from build123d import *

# Parameters (mm, degrees)
SKETCH1_W            = 13
SKETCH1_H            = 5.75
BOSS_EXTRUDE1_DEPTH  = 2.5
SKETCH2_W            = 0.75
SKETCH2_H            = 0.5
BOSS_EXTRUDE2_DEPTH  = 4
CHAMFER1_SIZE        = 0.2
SKETCH4_R            = 1
CUT_EXTRUDE1_DEPTH   = 6
SKETCH5_W            = 2
SKETCH5_H            = 0.2
BOSS_EXTRUDE3_DEPTH  = 5.75
CHAMFER2_SIZE        = 0.2
SKETCH10_W           = 13.0002
SKETCH10_H           = 5.7502
BOSS_EXTRUDE8_DEPTH  = 3.75
SKETCH11_W           = 3.5
SKETCH11_H           = 2.3
BOSS_EXTRUDE9_DEPTH  = 0.5
SKETCH12_W           = 3.5
SKETCH12_H           = 2.3
BOSS_EXTRUDE10_DEPTH = 0.5
SKETCH13_W           = 1
SKETCH13_H           = 2.5
BOSS_EXTRUDE11_DEPTH = 1
FILLET2_RADIUS       = 0.5
FILLET2_LENGTH       = 2.5
SKETCH14_W           = 5
SKETCH14_H           = 4.5
CUT_EXTRUDE2_DEPTH   = 0.05
SKETCH15_R           = 0.15
CUT_EXTRUDE3_DEPTH   = 10
SKETCH16_W           = 0.75
SKETCH16_H           = 4
CUT_EXTRUDE4_DEPTH   = 1.2


with BuildPart() as part:
    # Sketch1 → Boss-Extrude1 (new body)
    with BuildSketch(Plane.XY):
        Rectangle(SKETCH1_W, SKETCH1_H)
    extrude(amount=BOSS_EXTRUDE1_DEPTH)

    # Sketch2 → Boss-Extrude2 (add)
    with BuildSketch(Plane(origin=(0, 0, 0), x_dir=(-1, 0, 0), z_dir=(0, 0, -1))):
        Rectangle(SKETCH2_W, SKETCH2_H)
        with Locations((-5, 0)):
            Rectangle(SKETCH2_W, SKETCH2_H)
        with Locations((5, 0)):
            Rectangle(SKETCH2_W, SKETCH2_H)
    extrude(amount=BOSS_EXTRUDE2_DEPTH)

    # Chamfer1
    chamfer1_edges = [part.edges().sort_by_distance(p)[0] for p in [
        (-0.375, 0, -4),
        (0.375, 0, -4),
        (4.625, 0, -4),
        (5.375, 0, -4),
        (-5.375, 0, -4),
        (-4.625, 0, -4),
    ]]
    chamfer(chamfer1_edges, length=CHAMFER1_SIZE)

    # Sketch4 → Cut-Extrude1 (cut)
    with BuildSketch(Plane(origin=(0, 2.875, 0), x_dir=(1, 0, 0), z_dir=(0, 1, 0))):
        with Locations(Location((-3.25, -1.25, 0), (0, 0, 270))):
            Circle(SKETCH4_R)
        with Locations(Location((3.25, -1.25, 0), (0, 0, 270))):
            Circle(SKETCH4_R)
    extrude(amount=-CUT_EXTRUDE1_DEPTH, mode=Mode.SUBTRACT)

    # Sketch5 → Boss-Extrude3 (add)
    with BuildSketch(Plane(origin=(0, 2.875, 0), x_dir=(1, 0, 0), z_dir=(0, 1, 0))):
        with Locations((-3.25, 0.1)):
            Rectangle(SKETCH5_W, SKETCH5_H)
        with Locations((3.25, 0.1)):
            Rectangle(SKETCH5_W, SKETCH5_H)
    extrude(amount=-BOSS_EXTRUDE3_DEPTH)

    # Chamfer2
    chamfer2_edges = [part.edges().sort_by_distance(p)[0] for p in [
        (4.25, 0, 0),
        (2.25, 0, 0),
        (-2.25, 0, 0),
        (-4.25, 0, 0),
    ]]
    chamfer(chamfer2_edges, length=CHAMFER2_SIZE - 0.0001)  # a hair under: the kernel refuses the full size

    # Sketch10 → Boss-Extrude8 (add)
    with BuildSketch(Plane.XY.offset(2.5)):
        Rectangle(SKETCH10_W, SKETCH10_H)
    extrude(amount=BOSS_EXTRUDE8_DEPTH)

    # Sketch11 → Boss-Extrude9 (add)
    with BuildSketch(Plane.XZ.offset(2.8751)):
        with Locations((0, 1.35)):
            Rectangle(SKETCH11_W, SKETCH11_H)
    extrude(amount=-BOSS_EXTRUDE9_DEPTH)

    # Sketch12 → Boss-Extrude10 (add)
    with BuildSketch(Plane(origin=(0, 2.8751, 0), x_dir=(1, 0, 0), z_dir=(0, 1, 0))):
        with Locations((0, -1.35)):
            Rectangle(SKETCH12_W, SKETCH12_H)
    extrude(amount=-BOSS_EXTRUDE10_DEPTH)

    # Sketch13 → Boss-Extrude11 (add)
    with BuildSketch(Plane.XY.offset(6.25)):
        with Locations((-1.9999, 0)):
            Rectangle(SKETCH13_W, SKETCH13_H)
    extrude(amount=BOSS_EXTRUDE11_DEPTH)

    # Fillet2: full round fillet: the end face becomes a half cylinder, R = half its width
    fillet2_face = Plane((-1.9999, 0, 7.25), x_dir=(0, -1, 0), z_dir=(0, 0, 1))  # on the end face: x along it, z out of the body
    fillet2_slab = fillet2_face.offset(-FILLET2_RADIUS / 2) * Box(FILLET2_LENGTH, 2 * FILLET2_RADIUS, FILLET2_RADIUS, mode=Mode.PRIVATE)  # the body's end, R deep
    fillet2_round = Plane((-1.9999, 0, 6.75), x_dir=(0, 0, 1), z_dir=(0, -1, 0)) * Cylinder(FILLET2_RADIUS, FILLET2_LENGTH, mode=Mode.PRIVATE)  # its axis R under the face
    add(fillet2_slab - fillet2_round, mode=Mode.SUBTRACT)

    # Sketch14 → Cut-Extrude2 (cut)
    with BuildSketch(Plane.XY.offset(6.25)):
        with Locations((2.5001, 0)):
            Rectangle(SKETCH14_W, SKETCH14_H)
    extrude(amount=-CUT_EXTRUDE2_DEPTH, mode=Mode.SUBTRACT)

    # Sketch15 → Cut-Extrude3 (cut)
    with BuildSketch(Plane(origin=(0, 2.8751, 0), x_dir=(1, 0, 0), z_dir=(0, 1, 0))):
        with Locations(Location((-5.500093333, -5.75, 0), (0, 0, 270))):
            Circle(SKETCH15_R)
    extrude(amount=-CUT_EXTRUDE3_DEPTH, mode=Mode.SUBTRACT)

    # Sketch16 → Cut-Extrude4 (cut)
    with BuildSketch(Plane.XY.offset(6.25)):
        with Locations((-5.5001, 0)):
            Rectangle(SKETCH16_W, SKETCH16_H)
    extrude(amount=-CUT_EXTRUDE4_DEPTH, mode=Mode.SUBTRACT)


solid = part.part
The model under review builds one solid part; all positions refer to its coordinate system, in mm. A direction names the side the tool comes from. Round coordinates to 2 decimals unless told otherwise and drop trailing zeros. Order: outer loops, then holes, each group sorted by start corner. A loop starts at its lowest first (then second) coordinate and runs counter-clockwise, first axis right, second up. Notation, with made-up numbers: (46.25, 34) -> (81.25, 34) arc R24 ccw to (81.25, 70) -> close; hole circle Ø11 at (-32, 29.25). An arc over 180 degrees is marked (long way). Write item = value, one per line. Start each with the question number.
Item 1: Clearance check with flat-ended pins moving along their axes: pin 1 Ø0.6 at (y, z) = (0, -2.5) entering from +X (3 decimals); pin 2 Ø1.1 at (x, z) = (-2, 7) entering from +Y; pin 3 Ø1.5 at (x, y) = (4.5, -1) entering from +Z. State where each tip first meets the part, or that it passes through.
Item 2: Consider section D-D on z = 5.75. Write out the cut boundary in (x, y), plus the area to 3 significant figures.
Item 3: For faces 5 (the face through (4.24, 0.04, 1.12)), 6 (the face through (-5.875, 0, 6)), 7 (the face through (-2, -1.25, 7)), list the 3-axis set-ups (+Z, -Z, +X, -X, +Y, -Y) from which the entire face can be reached by the end or side of a thin tool; tool diameter is ignored.
Item 4: Consider section C-C on y = -1.55. Count the separate pieces of the cut face and the enclosed holes in it, plus the area to 3 significant figures.
Item 5: Mouldability with a two-part tool opening along X and no side actions: class faces 1 (the face through (-5.125, 0, 6)), 2 (the face through (0, 1, 0)), 3 (the face through (0, 2.875, 4)), 4 (the face through (-1.99, -0.02, 7.25)) as released by +X, released by -X, zero draft, split by the parting line, or undercut.
Item 6: For line 1 along X through (y, z) = (-0.9, 1.25); line 2 along X through (y, z) = (0.15, -2.5) (3 decimals); line 3 along X through (y, z) = (-2.45, 5.75), list the stretches that pass through material, from the lowest coordinate up.
Item 7: Consider section A-A on z = -0.5. Write out the cut boundary in (x, y) (3 decimals).
Conclusion:
q1.pin_1 = 5.375
q1.pin_2 = 1.25
q1.pin_3 = 6.25
q2.outline = (-6.5, -2.88) -> (-5.65, -2.88) -> (-5.65, -2) -> (-5.88, -2) -> (-5.88, 2) -> (-5.65, 2) -> (-5.65, 2.88) -> (-6.5, 2.88) -> close; (-5.35, -2.88) -> (6.5, -2.88) -> (6.5, 2.88) -> (-5.35, 2.88) -> (-5.35, 2) -> (-5.13, 2) -> (-5.13, -2) -> (-5.35, -2) -> close
q2.area = 71.2 mm2
q3.face_5 = +Y, -Y
q3.face_6 = +Z
q3.face_7 = +Z, +X, -X, -Y
q4.separate_pieces = 1
q4.enclosed_holes = 2
q4.area = 74.7 mm2
q5.face_1 = undercut
q5.face_2 = undercut
q5.face_3 = zero draft
q5.face_4 = split by the parting line
q6.line_1 = -6.5 to -4.25, -2.25 to 2.25, 4.25 to 6.5
q6.line_2 = -5.375 to -4.625, -0.375 to 0.375, 4.625 to 5.375
q6.line_3 = -6.5 to -5.65, -5.35 to 6.5
q7.outline = (-5.375, -0.25) -> (-4.625, -0.25) -> (-4.625, 0.25) -> (-5.375, 0.25) -> close; (-0.375, -0.25) -> (0.375, -0.25) -> (0.375, 0.25) -> (-0.375, 0.25) -> close; (4.625, -0.25) -> (5.375, -0.25) -> (5.375, 0.25) -> (4.625, 0.25) -> close
